Design review of the part shown in the three views and the two pictorial views. Dimensions are in mm from the part's minimum x, y and z. A direction names the side the tool comes from. Give positions to 0.01 mm unless a question says otherwise; leave off trailing zeros. Order: outer loops, then holes, each group sorted by start corner. A loop starts at its lowest first (then second) coordinate and runs counter-clockwise, first axis right, second up.
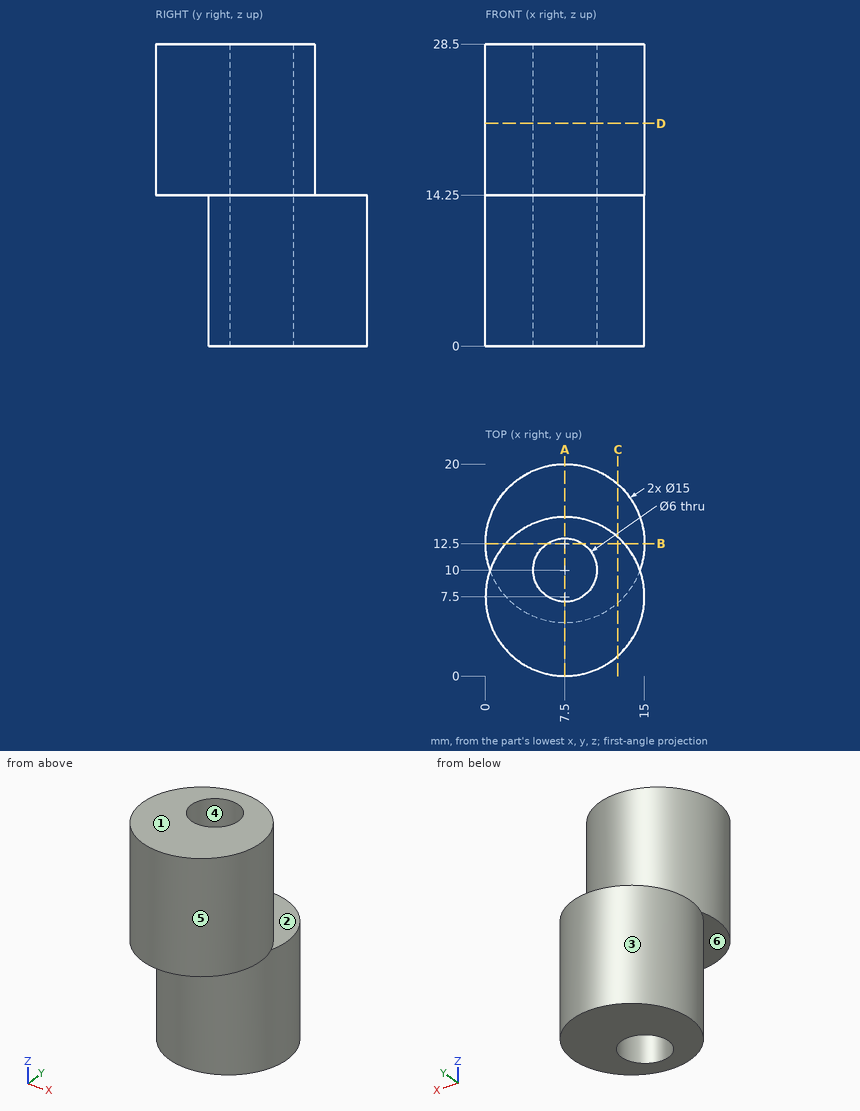
1) We need section D-D on z = 21. Give the boundary of the cut face in (x, y).
Answer sheet:
outline: circle Ø15 at (7.5, 7.5); hole circle Ø6 at (7.5, 10)
2) Clearance check with flat-ended pins moving along their axes: pin 1 (1 mm diameter, centred on x = 10.5, z = 19, fed in from +Y); pin 2 (1.5 mm diameter, centred on y = 4, z = 16.5, fed in from -X); pin 3 (3 mm diameter, centred on y = 17.5, z = 5, fed in from +X). State where each tip first meets the part, or that it passes through.
Answer sheet:
pin 1: stops at y = 14.57
pin 2: stops at x = 0.52
pin 3: stops at x = 14.13
3) Tool access review of the marked faces 1, 2 and 3: name each direction out of +Z, -Z, +X, -X, +Y, -Y from which nothing blocks a thin tool from reaching the whole face with its end or side.
Answer sheet:
face 1: +Z, +X, -X, +Y, -Y
face 2: +Z, +Y
face 3: -Z
4) We need section A-A on x = 7.5. Give the boundary of the cut face in (y, z), then the cut area to 4 significant figures.
Answer sheet:
outline: (0, 14.25) - (5, 14.25) - (5, 0) - (7, 0) - (7, 28.5) - (0, 28.5) - close; (13, 0) - (20, 0) - (20, 14.25) - (15, 14.25) - (15, 28.5) - (13, 28.5) - close
area: 256.5 mm2
5) We need section C-C on x = 12.5. Give the boundary of the cut face in (y, z).
Answer sheet:
outline: (1.91, 14.25) - (6.91, 14.25) - (6.91, 0) - (18.09, 0) - (18.09, 14.25) - (13.09, 14.25) - (13.09, 28.5) - (1.91, 28.5) - close
6) Draft analysis for pull direction Y (two halves, no side actions). For the marked faces 4, 5 and 6, state which applies: +Y half, -Y half, draft (parallel to the pull), parting line (faces both ways), or undercut.
Answer sheet:
face 4: undercut
face 5: parting line
face 6: draft
7) We need section B-B on y = 12.5. Give the boundary of the cut face in (x, z).
Answer sheet:
outline: (0, 0) - (5.84, 0) - (5.84, 28.5) - (1.91, 28.5) - (1.91, 14.25) - (0, 14.25) - close; (9.16, 0) - (15, 0) - (15, 14.25) - (13.09, 14.25) - (13.09, 28.5) - (9.16, 28.5) - close
8) To check wall thickness, follow line 1 (Y direction, x = 7.5, z = 12); line 2 (Z direction, x = 6, y = 15.75); line 3 (Y direction, x = 6.75, z = 25.75). State the ranges of each line that lie inside material, in increasing order.
Answer sheet:
line 1: y = 5 to 7, 13 to 20
line 2: z = 0 to 14.25
line 3: y = 0.04 to 7.1, 12.9 to 14.96
